Build history of the part. All positions in model axes, mm. A direction names the side the tool comes from. Round coordinates to 2 decimals unless told otherwise and drop trailing zeros. Loops run counter-clockwise (first coordinate to the right, second up) from the corner with the lowest first, then second, coordinate; pieces in that order, holes last.
from build123d import *

# Parameters (mm, degrees)
SKETCH_1_W                      = 53
SKETCH_1_H                      = 32
EXTRUDE_1_DEPTH                 = 2
SKETCH_1_5_W                    = 0.8
SKETCH_1_5_H                    = 32
EXTRUDE_3_DEPTH                 = 0.8
SKETCH_1_6_W                    = 0.8
SKETCH_1_6_H                    = 32
EXTRUDE_4_DEPTH                 = 0.8
SKETCH_3_W                      = 54.6
SKETCH_3_H                      = 1
EXTRUDE_5_DEPTH                 = 0.8
SKETCH_4_W                      = 45
SKETCH_4_H                      = 1
CUT_EXTRUDE_1_DEPTH             = 33.222507662
SKETCH_4_2_W                    = 45
SKETCH_4_2_H                    = 1
EXTRUDE_6_DEPTH                 = 2
SKETCH_5_W                      = 45
SKETCH_5_H                      = 1
CUT_EXTRUDE_2_DEPTH             = 2
SKETCH_6_W                      = 0.8
SKETCH_6_H                      = 1
CUT_EXTRUDE_3_DEPTH             = 10
EXTRUDE_7_DEPTH                 = 18
EXTRUDE_7_DEPTH_BACK            = 12
EXTRUDE_8_DEPTH                 = 18
EXTRUDE_8_DEPTH_BACK            = 12
SKETCH_8_W                      = 49
SKETCH_8_H                      = 2
CUT_EXTRUDE_4_REACH             = 39.802
SKETCH_12_W                     = 2
SKETCH_12_H                     = 0.755050506
CUT_EXTRUDE_4_DIRECTION_2_REACH = 39.802
CUT_EXTRUDE_5_REACH             = 48.787
SKETCH_9_W                      = 48.171487548
SKETCH_9_H                      = 25.213726265
CUT_EXTRUDE_6_REACH             = 48.787
SKETCH_13_W                     = 1
SKETCH_13_H                     = 0.8
SKETCH_14_W                     = 8
SKETCH_14_H                     = 12
EXTRUDE_9_DEPTH                 = 18


with BuildPart() as part:
    # 草图1 → 凸台-拉伸1 (new body)
    with BuildSketch(Plane(origin=(0, 0, 0), x_dir=(1, 0, 0), z_dir=(0, 1, 0))):
        Rectangle(SKETCH_1_W, SKETCH_1_H)
    extrude(amount=EXTRUDE_1_DEPTH)

    # 草图1<5> → 凸台-拉伸3 (add)
    with BuildSketch(Plane(origin=(0, 0, 0), x_dir=(1, 0, 0), z_dir=(0, 1, 0))):
        with Locations((-26.9, 0)):
            Rectangle(SKETCH_1_5_W, SKETCH_1_5_H)
    extrude(amount=EXTRUDE_3_DEPTH)

    # 草图1<6> → 凸台-拉伸4 (add)
    with BuildSketch(Plane(origin=(0, 0, 0), x_dir=(1, 0, 0), z_dir=(0, 1, 0))):
        with Locations((26.9, 0)):
            Rectangle(SKETCH_1_6_W, SKETCH_1_6_H)
    extrude(amount=EXTRUDE_4_DEPTH)

    # 草图3 → 凸台-拉伸5 (add)
    with BuildSketch(Plane(origin=(0, 0, 0), x_dir=(1, 0, 0), z_dir=(0, 1, 0))):
        with Locations((0, -16.5)):
            Rectangle(SKETCH_3_W, SKETCH_3_H)
    extrude(amount=EXTRUDE_5_DEPTH)

    # 草图4 → 切除-拉伸1 (cut, through all)
    with BuildSketch(Plane(origin=(0, 0, 0), x_dir=(1, 0, 0), z_dir=(0, 1, 0))):
        with Locations((0, -14.5)):
            Rectangle(SKETCH_4_W, SKETCH_4_H)
    extrude(amount=CUT_EXTRUDE_1_DEPTH, mode=Mode.SUBTRACT)

    # 草图4<2> → 凸台-拉伸6 (add)
    with BuildSketch(Plane(origin=(0, 0, 0), x_dir=(1, 0, 0), z_dir=(0, 1, 0))):
        with Locations((0, -14.5)):
            Rectangle(SKETCH_4_2_W, SKETCH_4_2_H)
    extrude(amount=EXTRUDE_6_DEPTH)

    # 草图5 → 切除-拉伸2 (cut)
    with BuildSketch(Plane(origin=(0, 0, 0), x_dir=(1, 0, 0), z_dir=(0, 1, 0))):
        with Locations((0, 14.5)):
            Rectangle(SKETCH_5_W, SKETCH_5_H)
    extrude(amount=CUT_EXTRUDE_2_DEPTH, mode=Mode.SUBTRACT)

    # 草图6 → 切除-拉伸3 (cut)
    with BuildSketch(Plane(origin=(0, 0, 0), x_dir=(1, 0, 0), z_dir=(0, 1, 0))):
        with Locations((-26.9, -16.5)):
            Rectangle(SKETCH_6_W, SKETCH_6_H)
        with Locations((26.9, -16.5)):
            Rectangle(SKETCH_6_W, SKETCH_6_H)
    extrude(amount=CUT_EXTRUDE_3_DEPTH, mode=Mode.SUBTRACT)

    # 草图7 → 凸台-拉伸7 (add, two sides: drawn at the far end of the back side and taken through both)
    with BuildSketch(Plane.XY.offset(-EXTRUDE_7_DEPTH_BACK)):
        Polygon((-24.5, 2), (-24.5, 4), (-33, 4), (-33, -1), (-31, -1), (-31, 2), align=None)
        Polygon((24.5, 2), (24.5, 4), (33, 4), (33, -1), (31, -1), (31, 2), align=None)
    extrude(amount=EXTRUDE_7_DEPTH + EXTRUDE_7_DEPTH_BACK)

    # 草图8 → 凸台-拉伸8 (add, two sides: drawn at the far end of the back side and taken through both)
    with BuildSketch(Plane.XY.offset(-EXTRUDE_8_DEPTH_BACK)):
        with Locations((0, 3)):
            Rectangle(SKETCH_8_W, SKETCH_8_H)
    extrude(amount=EXTRUDE_8_DEPTH + EXTRUDE_8_DEPTH_BACK)

    # 切除-拉伸4: up to this face of the body (flat: up to its plane)
    cut_extrude_4_end = Plane(part.part.faces().sort_by_distance((-31, 0.5, 3))[0])
    # 草图12 → 切除-拉伸4 (cut, up to the picked face)
    with BuildSketch(Plane(origin=(0, 0, 0), x_dir=(0, 0, -1), z_dir=(1, 0, 0)), mode=Mode.PRIVATE) as cut_extrude_4_sk1:
        with Locations((-17, 2.377525253)):
            Rectangle(SKETCH_12_W, SKETCH_12_H)
    cut_extrude_4_tool1 = split(extrude(cut_extrude_4_sk1.sketch, amount=-CUT_EXTRUDE_4_REACH, mode=Mode.PRIVATE), bisect_by=cut_extrude_4_end, keep=Keep.BOTH, mode=Mode.PRIVATE)
    add(cut_extrude_4_tool1.solids().sort_by(Axis((0, 2.377525, 17), (-1, 0, 0)))[0], mode=Mode.SUBTRACT)

    # 切除-拉伸4 direction 2: up to this face of the body (flat: up to its plane)
    cut_extrude_4_direction_2_end = Plane(part.part.faces().sort_by_distance((31, 0.5, 3))[0])
    # 草图12 → 切除-拉伸4 direction 2 (cut, up to the picked face)
    with BuildSketch(Plane(origin=(0, 0, 0), x_dir=(0, 0, -1), z_dir=(1, 0, 0)), mode=Mode.PRIVATE) as cut_extrude_4_direction_2_sk1:
        with Locations((-17, 2.377525253)):
            Rectangle(SKETCH_12_W, SKETCH_12_H)
    cut_extrude_4_direction_2_tool1 = split(extrude(cut_extrude_4_direction_2_sk1.sketch, amount=CUT_EXTRUDE_4_DIRECTION_2_REACH, mode=Mode.PRIVATE), bisect_by=cut_extrude_4_direction_2_end, keep=Keep.BOTH, mode=Mode.PRIVATE)
    add(cut_extrude_4_direction_2_tool1.solids().sort_by(Axis((0, 2.377525, 17), (1, 0, 0)))[0], mode=Mode.SUBTRACT)

    # 草图9 → 切除-拉伸5 (cut, up to next)
    with BuildSketch(Plane(origin=(10, 0, 0), x_dir=(0, 0, -1), z_dir=(1, 0, 0)), mode=Mode.PRIVATE) as cut_extrude_5_sk1:
        with Locations((-3.488196671, 1.118476511)):
            Rectangle(SKETCH_9_W, SKETCH_9_H)
    cut_extrude_5_tool1 = extrude(cut_extrude_5_sk1.sketch, amount=CUT_EXTRUDE_5_REACH, mode=Mode.PRIVATE) & part.part
    add(cut_extrude_5_tool1.solids().sort_by_distance((10, 1.118477, 3.488197))[0], mode=Mode.SUBTRACT)

    # 草图13 → 切除-拉伸6 (cut, up to next)
    with BuildSketch(Plane(origin=(10, 0, 0), x_dir=(0, 0, -1), z_dir=(1, 0, 0)), mode=Mode.PRIVATE) as cut_extrude_6_sk1:
        with Locations((-16.5, 0.4)):
            Rectangle(SKETCH_13_W, SKETCH_13_H)
    cut_extrude_6_tool1 = extrude(cut_extrude_6_sk1.sketch, amount=-CUT_EXTRUDE_6_REACH, mode=Mode.PRIVATE) & part.part
    add(cut_extrude_6_tool1.solids().sort_by_distance((10, 0.4, 16.5))[0], mode=Mode.SUBTRACT)

    # 草图14 → 凸台-拉伸9 (add, through all)
    with BuildSketch(Plane.XY):
        with Locations((-18.5, 10)):
            Rectangle(SKETCH_14_W, SKETCH_14_H)
    extrude(amount=EXTRUDE_9_DEPTH)


solid = part.part
(1) Pin check, flat tips, straight feed: P1, Ø10, axis at x = -10.5, y = 13, coming from the -Z side; P2, Ø6.5, axis at x = -17.5, y = 7, coming from the -Z side; P3, Ø9.5, axis at y = 12, z = 8, coming from the +X side. Stop position of each tip, or through.
Responses:
P1: stops at z = 0
P2: stops at z = -12
P3: stops at x = -14.5
(2) Slice it at A-A on x = -5. List the corners of the cut face in (y, z), plus the area to 3 significant figures.
Responses:
outline: (0, -16) - (2, -16) - (2, -15) - (0, -15) - close; (0, -14) - (2, -14) - (2, -12) - (4, -12) - (4, 18) - (2.76, 18) - (2.76, 16) - (0, 16) - close
area: 120 mm2
(3) Slice it at D-D on x = -17.5. List the corners of the cut face in (y, z), plus the area to 3 significant figures.
Responses:
outline: (0, -16) - (2, -16) - (2, -15) - (0, -15) - close; (0, -14) - (2, -14) - (2, -12) - (4, -12) - (4, 0) - (16, 0) - (16, 18) - (2.76, 18) - (2.76, 16) - (0, 16) - close
area: 336 mm2
(4) Slice it at C-C on x = -26. List the corners of the cut face in (y, z).
Responses:
outline: (0, -16) - (2, -16) - (2, -12) - (4, -12) - (4, 18) - (2.76, 18) - (2.76, 16) - (0, 16) - close
(5) Probe line 1 (X direction, y = 0.5, z = 3.5); line 2 (Z direction, x = -25.5, y = 0.5); line 3 (Y direction, x = 5.5, z = -10). List the from-to ranges inside material, lowest first.
Responses:
line 1: x = -33 to -31, -27.3 to 10
line 2: z = -16 to 16
line 3: y = 0 to 4
(6) Slice it at B-B on z = -5. List the corners of the cut face in (x, y).
Responses:
outline: (-33, -1) - (-31, -1) - (-31, 2) - (-26.5, 2) - (-26.5, 0.8) - (-27.3, 0.8) - (-27.3, 0) - (10, 0) - (10, 4) - (-33, 4) - close
(7) Pull direction X, two halves, no side cores. Call faces 4 (the face through (-22.5, 1, -14.5)), 5 (the face through (-19, 16, 9)), 6 (the face through (-31, 0, 3)), 7 (the face through (-22.5, 10, 9)): +X half, -X half, draft (parallel to the pull), parting line (faces both ways), or undercut.
Responses:
face 4: +X half
face 5: draft
face 6: undercut
face 7: -X half
(8) Which spindle directions (+Z, -Z, +X, -X, +Y, -Y) get a long thin tool onto all of the face, cutting with end or side? Do faces 1 (the face through (-6, 1, -15)), 2 (the face through (-9, 0, 0)), 3 (the face through (-26.5, 1, 0)). Say none if no direction does.
Responses:
face 1: +X, +Y, -Y
face 2: +Z, -Z, +X, -Y
face 3: +Z, -Z
